from build123d import *

# Parameters (mm, degrees)
SALIENTE_EXTRUIR1_DEPTH = 30
CORTAR_EXTRUIR2_DEPTH   = 90
CROQUIS5_W              = 20
CROQUIS5_H              = 2
SALIENTE_EXTRUIR2_DEPTH = 3
CHAFL_N1_SIZE           = 15
CHAFL_N1_SIZE2          = 4.585960222
CHAFL_N2_SIZE           = 15
CHAFL_N2_SIZE2          = 4.585960222
CHAFL_N3_SIZE           = 15
CHAFL_N3_SIZE2          = 4.873795443


with BuildPart() as part:
    # Croquis2 → Saliente-Extruir1 (new body)
    with BuildSketch(Plane(origin=(0, 0, 0), x_dir=(1, 0, 0), z_dir=(0, 1, 0))):
        Polygon((4.293050572, 35.408576274), (-0.206949428, 35.33296049), (-14, 0), (0, 0), (3.44434788, 28.408576274), align=None)
        Polygon((45.293050572, 35.408576274), (4.293050572, 35.408576274), (3.44434788, 28.408576274), (46.141753264, 28.408576274), align=None)
        Polygon((49.793050572, 35.33296049), (45.293050572, 35.408576274), (46.141753264, 28.408576274), (49.586101144, 0), (63.586101144, 0), align=None)
    extrude(amount=SALIENTE_EXTRUIR1_DEPTH)

    # Croquis4 → Cortar-Extruir2 (cut, symmetric)
    with BuildSketch(Plane(origin=(0, 0, 0), x_dir=(0, 0, -1), z_dir=(1, 0, 0))):
        Polygon((0, 0), (5, 0), (5, 30), (-4.90661078, 30), (-4.90661078, 0), align=None)
    extrude(amount=CORTAR_EXTRUIR2_DEPTH, both=True, mode=Mode.SUBTRACT)

    # Croquis5 → Saliente-Extruir2 (add)
    with BuildSketch(Plane(origin=(0, 0, 0), x_dir=(-1, 0, 0), z_dir=(0, -1, 0))):
        with Locations((-24.793050572, 32.408576274)):
            Rectangle(CROQUIS5_W, CROQUIS5_H)
    extrude(amount=SALIENTE_EXTRUIR2_DEPTH)

    # Chaflán1
    chafl_n1_edges = [part.edges().sort_by_distance(p)[0] for p in [
        (2.025282044, 30, -16.704288137),
    ]]
    chafl_n1_side = [part.faces().sort_by_distance(p)[0] for p in [
        (2.025282044, 15, -16.704288137),
    ]]
    chamfer(chafl_n1_edges, length=CHAFL_N1_SIZE, length2=CHAFL_N1_SIZE2, reference=chafl_n1_side[0])

    # Chaflán2
    chafl_n2_edges = [part.edges().sort_by_distance(p)[0] for p in [
        (47.5608191, 30, -16.704288137),
    ]]
    chafl_n2_side = [part.faces().sort_by_distance(p)[0] for p in [
        (47.5608191, 15, -16.704288137),
    ]]
    chamfer(chafl_n2_edges, length=CHAFL_N2_SIZE, length2=CHAFL_N2_SIZE2, reference=chafl_n2_side[0])

    # Chaflán3
    chafl_n3_edges = [part.edges().sort_by_distance(p)[0] for p in [
        (24.793050572, 30, -28.408576274),
    ]]
    chafl_n3_side = [part.faces().sort_by_distance(p)[0] for p in [
        (24.793050572, 15.5132008, -28.408576274),
    ]]
    chamfer(chafl_n3_edges, length=CHAFL_N3_SIZE, length2=CHAFL_N3_SIZE2, reference=chafl_n3_side[0])


solid = part.part
Could you check a few things on this model? Use its own coordinates, in mm. A direction names the side the tool comes from. Round coordinates to 2 decimals unless told otherwise and drop trailing zeros. Loops run counter-clockwise (first coordinate to the right, second up) from the corner with the lowest first, then second, coordinate; pieces in that order, holes last. Notation, with made-up numbers: (84.5, 69.5) - (114.5, 69.5) arc R21 ccw to (114.5, 91.5) - close; hole circle Ø6 at (11, 3.25). An arc over 180 degrees is marked (long way). Write item = value, one per line.
1) Imagine slicing it at D-D (z = -20). Please give me the cut outline in (x, y), and give its area (3 significant figures).
Computed:
outline = (-6.19, 0) - (2.42, 0) - (2.42, 15) - (-2.19, 30) - (-6.19, 30) - close; (47.16, 0) - (55.78, 0) - (55.78, 30) - (51.78, 30) - (47.16, 15) - close
area = 448 mm2
2) Imagine slicing it at B-B (x = 24). Please give me the cut outline in (y, z).
Computed:
outline = (-3, -33.41) - (0, -33.41) - (0, -35.41) - (30, -35.41) - (30, -33.28) - (15, -28.41) - (0, -28.41) - (0, -31.41) - (-3, -31.41) - close
3) I need wall thicknesses on line 1 along X through (y, z) = (22, -26.5); line 2 along Y through (x, z) = (-4, -20); line 3 along Z through (x, y) = (38.5, 4.5). Which ranges of each line are inside material? Lowest first, please. Write a range as from..to.
Computed:
line_1 = -3.66..1.06, 48.53..53.24
line_2 = 0..30
line_3 = -35.41..-28.41
4) Imagine slicing it at C-C (y = 5.5). Please give me the cut outline in (x, z).
Computed:
outline = (-12.05, -5) - (-0.21, -35.33) - (4.29, -35.41) - (45.29, -35.41) - (49.79, -35.33) - (61.63, -5) - (48.98, -5) - (46.14, -28.41) - (3.44, -28.41) - (0.61, -5) - close
5) I'm going to push flat-ended pins straight in: P1, Ø3, axis at y = 15, z = -14, coming from the +X side; P2, Ø4.5, axis at x = 18, y = 7, coming from the +Z side; P3, Ø2.5, axis at x = 27.5, y = -1.5, coming from the -Z side. Where does each tip first touch, or does it pass through?
Computed:
P1 = 58.71
P2 = -28.41
P3 = -33.41
6) Imagine slicing it at A-A (z = -15). Please give me the cut outline in (x, y).
Computed:
outline = (-8.14, 0) - (1.82, 0) - (1.82, 15) - (-2.8, 30) - (-8.14, 30) - close; (47.77, 0) - (57.73, 0) - (57.73, 30) - (52.39, 30) - (47.77, 15) - close
7) On a 3-axis mill with a long thin cutter (end or side, diameter ignored), from which of +Z, -Z, +X, -X, +Y, -Y can I reach the whole of each face in a straight line? I mean faces 4 (the flat face through (14.793, -1, -32)), 5 (the flat face through (24.44, 22.61, -30.88)), 6 (the flat face through (24, 7, -28.409)), 7 (the flat face through (25, -1, -33.409)). Say none if no direction works.
Computed:
face_4 = +Z, -Z, -X, -Y
face_5 = +Z, +Y
face_6 = +Z, +Y, -Y
face_7 = -Z, +X, -X, -Y
8) If we mould it in two halves opening along X, with no side actions, what happens to faces 1 (the flat face through (-0.08, 22.61, -18.67)), 2 (the flat face through (-6.045, 14.79, -20.379)), 3 (the flat face through (-6, 15, -5))? For each: pulls with the +X half, pulls with the -X half, needs draft (parallel to the pull), parting line crosses it, or undercut.
Computed:
face_1 = undercut
face_2 = pulls with the -X half
face_3 = needs draft
